Model file for the job. Use its own axes, mm. A direction names the side the tool comes from. Round coordinates to 2 decimals unless told otherwise and drop trailing zeros. Loops run counter-clockwise (first coordinate to the right, second up) from the corner with the lowest first, then second, coordinate; pieces in that order, holes last. Notation, with made-up numbers: M -26.75,-9.75 L -10.75,-9.75 A30 cw -10.75,21.25 Z; hole C 68,-36 d8. An arc over 180 degrees is marked long. Use a Markdown table: item, result. Add a question column.
Q1. Probe line 1 (Z direction, x = 0, y = 71); line 2 (X direction, y = 36.5, z = 0); line 3 (Z direction, x = 0, y = 34.5). List the from-to ranges inside material, lowest first. Write a range as from..to.
Q2. Cut at C-C (x = 53). State how many separate pieces and enclosed holes the cut face has, plus the area to 3 significant figures.
Q3. Cut at A-A (y = 71.5). Give the cut face in (x, z).
Q4. Cut at B-B (z = -59). Give the cut face in (x, y).
Q5. Tool access for faces 1 (the face through (2.1, 18, -25.1)), 2 (the face through (-17.35, 59.24, 29.33)), 3 (the face through (31, 59, 0)), 4 (the face through (-45.59, 7, -30.79)): list every direction of +Z, -Z, +X, -X, +Y, -Y with a clear straight run to the whole face (end or side of a thin tool).
Q6. Pin check, flat tips, straight feed: pin 1 (9 mm diameter, centred on x = 50.5, z = -31, fed in from +Y); pin 2 (1.5 mm diameter, centred on x = -27.5, y = 57, fed in from +Z); pin 3 (8 mm diameter, centred on x = 47.5, z = 0, fed in from +Y). Stop position of each tip, or through.
Q7. Mould opens along Z. For faces 5 (the face through (-31, 59, 0)), 6 (the face through (-46.235, 29.339, 16.238)), 7 (the face through (-56.465, 3.451, -28.308)), 8 (the face through (-17.119, 59.241, -29.665)) say: +Z half, -Z half, draft (parallel to the pull), parting line (faces both ways), or undercut.
from build123d import *

# Parameters (mm, degrees)
SKETCH1_R                               = 71
BOSS_EXTRUDE1_DEPTH                     = 18
BOSS_EXTRUDE2_DEPTH                     = 23
BOSS_EXTRUDE3_DEPTH                     = 37
CBORE_FOR_M5_HEX_HEAD_BOLT1_D           = 11
CBORE_FOR_M5_HEX_HEAD_BOLT1_CBORE_D     = 18
CBORE_FOR_M5_HEX_HEAD_BOLT1_CBORE_DEPTH = 11
CIRPATTERN1_COUNT                       = 6
F_10_0MM_DOWEL_HOLE1_D                  = 10
F_10_0MM_DOWEL_HOLE1_DEPTH              = 15
F_10_0MM_DOWEL_HOLE1_TIP                = 3.004303095
MIRROR2_OUTLINE_W                       = 2.5
MIRROR2_OUTLINE_H                       = 12.566951185
CUT_EXTRUDE1_REACH                      = 110.457
SKETCH17_R                              = 2.5


# Read off the part's stored shape, not the designer's step: Mirror2
with BuildPart() as part:
    # Sketch1 → Boss-Extrude1 (new body)
    with BuildSketch(Plane(origin=(0, 0, 0), x_dir=(1, 0, 0), z_dir=(0, 1, 0))):
        with Locations(Location((0, 0, 0), (0, 0, 270))):
            Circle(SKETCH1_R)
    extrude(amount=BOSS_EXTRUDE1_DEPTH)

    # Sketch2 → Boss-Extrude2 (add)
    with BuildSketch(Plane(origin=(0, 18, 0), x_dir=(1, 0, 0), z_dir=(0, 1, 0))):
        with BuildLine():
            Line((-50.50990002, 15), (-69.397406292, 15))
            ThreePointArc((-69.397406292, 15), (-71, 0), (-69.397406292, -15))
            Line((-69.397406292, -15), (-50.50990002, -15))
            ThreePointArc((-50.50990002, -15), (-46.181073535, -16.272350986), (-43.229193711, -19.684684685))
            ThreePointArc((-43.229193711, -19.684684685), (0, -47.5), (43.229193711, -19.684684685))
            ThreePointArc((43.229193711, -19.684684685), (46.181073535, -16.272350986), (50.50990002, -15))
            Line((50.50990002, -15), (69.397406292, -15))
            ThreePointArc((69.397406292, -15), (71, 0), (69.397406292, 15))
            Line((69.397406292, 15), (50.50990002, 15))
            ThreePointArc((50.50990002, 15), (46.181073535, 16.272350986), (43.229193711, 19.684684685))
            ThreePointArc((43.229193711, 19.684684685), (0, 47.5), (-43.229193711, 19.684684685))
            ThreePointArc((-43.229193711, 19.684684685), (-46.181073535, 16.272350986), (-50.50990002, 15))
        make_face()
    extrude(amount=BOSS_EXTRUDE2_DEPTH)

    # Sketch3 → Boss-Extrude3 (add)
    with BuildSketch(Plane(origin=(0, 41, 0), x_dir=(1, 0, 0), z_dir=(0, 1, 0))):
        with BuildLine():
            Line((9.027169873, -41.285714286), (25.440206006, -17.714285714))
            ThreePointArc((25.440206006, -17.714285714), (31, 0), (25.440206006, 17.714285714))
            Line((25.440206006, 17.714285714), (9.027169873, 41.285714286))
            ThreePointArc((9.027169873, 41.285714286), (0, 46), (-9.027169873, 41.285714286))
            Line((-9.027169873, 41.285714286), (-25.440206006, 17.714285714))
            ThreePointArc((-25.440206006, 17.714285714), (-31, 0), (-25.440206006, -17.714285714))
            Line((-25.440206006, -17.714285714), (-9.027169873, -41.285714286))
            ThreePointArc((-9.027169873, -41.285714286), (0, -46), (9.027169873, -41.285714286))
        make_face()
    extrude(amount=BOSS_EXTRUDE3_DEPTH)

    # CBORE for M5 Hex Head Bolt1 (through all)
    with Locations(Plane(origin=(0, 18, 59), x_dir=(0, 0, 1), z_dir=(0, 1, 0))):
        with Locations((0, 0)):
            cbore_for_m5_hex_head_bolt1 = CounterBoreHole(CBORE_FOR_M5_HEX_HEAD_BOLT1_D / 2, CBORE_FOR_M5_HEX_HEAD_BOLT1_CBORE_D / 2, CBORE_FOR_M5_HEX_HEAD_BOLT1_CBORE_DEPTH)

    # CirPattern1: CBORE for M5 Hex Head Bolt1 ×6 about axis
    cirpattern1_axis = Axis((0, 0, 0), (0, 1, 0))
    for i in range(1, CIRPATTERN1_COUNT):
        add(cbore_for_m5_hex_head_bolt1.rotate(cirpattern1_axis, i * 360 / CIRPATTERN1_COUNT), mode=Mode.SUBTRACT)

    # Ø10.0mm Dowel Hole1
    with Locations(Plane(origin=(0, 78, -35), x_dir=(0, 0, 1), z_dir=(0, 1, 0))):
        with Locations((0, 0), (70, 0)):
            Hole(F_10_0MM_DOWEL_HOLE1_D / 2, depth=F_10_0MM_DOWEL_HOLE1_DEPTH)
            with Locations((0, 0, -(F_10_0MM_DOWEL_HOLE1_DEPTH + F_10_0MM_DOWEL_HOLE1_TIP / 2))):  # 118° drill point
                Cone(0, F_10_0MM_DOWEL_HOLE1_D / 2, F_10_0MM_DOWEL_HOLE1_TIP, mode=Mode.SUBTRACT)

    # Sketch12 → Cut-Revolve3 (revolve, cut)
    with BuildSketch(Plane(origin=(0, 0, 0), x_dir=(0, 0, -1), z_dir=(1, 0, 0))):
        with BuildLine():
            Line((0, 0), (31, 0))
            Line((31, 0), (31, 18))
            Line((31, 18), (25, 18))
            Line((25, 18), (22.043106659, 29.03527618))
            ThreePointArc((22.043106659, 29.03527618), (20.61444907, 31.173413361), (18.179403354, 32))
            Line((18.179403354, 32), (11.248711306, 32))
            Line((11.248711306, 32), (11.248711306, 41))
            Line((11.248711306, 41), (23, 41))
            Line((23, 41), (23, 78))
            Line((23, 78), (0, 78))
            Line((0, 78), (0, 0))
        make_face()
    revolve(axis=Axis((0, 0, 0), (0, 1, 0)), mode=Mode.SUBTRACT)

    # Sketch13 → CBORE for M5 Hex Head Bolt2 (revolve, cut)
    with BuildSketch(Plane(origin=(-70.999948097, 18, -0.085850351), x_dir=(-0.001209159868286979, 0, 0.9999992689659393), z_dir=(0, 1, 0))):
        Polygon((0, 0), (0, 35.605163714), (6, 32), (6, 4), (10, 4), (10, 0), align=None)
    cbore_for_m5_hex_head_bolt2 = revolve(axis=Axis((-77.349943455, 18, -0.093528516), (0.9999992689659393, 0, 0.001209159868286979)), mode=Mode.SUBTRACT)

    # Mirror1: CBORE for M5 Hex Head Bolt2 across plane
    add(cbore_for_m5_hex_head_bolt2.mirror(Plane(origin=(0, 0, 0), x_dir=(0, 0, 1), z_dir=(1, 0, 0))), mode=Mode.SUBTRACT)

    # Sketch16 → Ø5.0mm Dowel Hole1 (revolve, cut)
    with BuildSketch(Plane(origin=(-70.999948097, 18, -0.085850351), x_dir=(-0.001209159868286979, 0, 0.9999992689659393), z_dir=(0, 1, 0))):
        Polygon((0, 0), (0, 72.501151548), (2.5, 70.999), (2.5, 0), align=None)
    revolve(axis=Axis((-77.349943455, 18, -0.093528516), (0.9999992689659393, 0, 0.001209159868286979)), mode=Mode.SUBTRACT)

    # Mirror2 outline → Mirror2 (revolve, cut)
    with BuildSketch(Plane(origin=(0, 18, 0), x_dir=(0, 1, 0), z_dir=(-0.0012091598682869803, 0, -0.9999992689659393))):
        with Locations((1.25, 30.613512241)):
            Rectangle(MIRROR2_OUTLINE_W, MIRROR2_OUTLINE_H)
        Polygon((2.5, -25.031211929), (2.5, -24.330096403), (2.439383393, -24.330096403), (2.439383393, -25.067634061), align=None)
    revolve(axis=Axis((0, 18, 0), (0.9999992689659393, 0, -0.0012091598682869803)), mode=Mode.SUBTRACT)

    # Sketch17 → Cut-Extrude1 (cut, up to next)
    with BuildSketch(Plane(origin=(0, 41, 0), x_dir=(1, 0, 0), z_dir=(0, 1, 0)), mode=Mode.PRIVATE) as cut_extrude1_sk1:
        with Locations(Location((-47.5, 0, 0), (0, 0, 270))):
            Circle(SKETCH17_R)
    cut_extrude1_tool1 = extrude(cut_extrude1_sk1.sketch, amount=-CUT_EXTRUDE1_REACH, mode=Mode.PRIVATE) & part.part
    # Sketch17 → Cut-Extrude1 (cut, up to next)
    with BuildSketch(Plane(origin=(0, 41, 0), x_dir=(1, 0, 0), z_dir=(0, 1, 0)), mode=Mode.PRIVATE) as cut_extrude1_sk2:
        with Locations(Location((47.5, 0, 0), (0, 0, 270))):
            Circle(SKETCH17_R)
    cut_extrude1_tool2 = extrude(cut_extrude1_sk2.sketch, amount=-CUT_EXTRUDE1_REACH, mode=Mode.PRIVATE) & part.part
    add(cut_extrude1_tool1.solids().sort_by_distance((-47.5, 41, 0))[0], mode=Mode.SUBTRACT)
    add(cut_extrude1_tool2.solids().sort_by_distance((47.5, 41, 0))[0], mode=Mode.SUBTRACT)


solid = part.part
Checked values:
| question | item | result |
|---|---|---|
| 1 | line 1 | z = -46..-40, -30..-23, 23..30, 40..46 |
| 1 | line 2 | x = -71..-50, -45..-11.25, 11.25..45, 50..71 |
| 1 | line 3 | z = -47.5..-11.25, 11.25..47.5 |
| 2 | separate pieces | 3 |
| 2 | enclosed holes | 1 |
| 2 | area | 1,750 mm^2 |
| 3 | outline | M -25.44,-17.71 L -9.03,-41.29 A11 ccw 9.03,-41.29 L 25.44,-17.71 A31 ccw 25.44,17.71 L 9.03,41.29 A11 ccw -9.03,41.29 L -25.44,17.71 A31 ccw Z; hole C 0,0 d46; hole C 0,-35 d10; hole C 0,35 d10 |
| 4 | outline | M -39.5,0 L -5.5,0 L -5.5,7 L -9,7 L -9,18 L -39.5,18 Z; M 5.5,0 L 39.5,0 L 39.5,18 L 9,18 L 9,7 L 5.5,7 Z |
| 5 | face 1 | -Y |
| 5 | face 2 | +Z, -X, +Y |
| 5 | face 3 | +X, +Y |
| 5 | face 4 | +Y |
| 6 | pin 1 | stops at y = 7 |
| 6 | pin 2 | stops at z = 15.67 |
| 6 | pin 3 | stops at y = 41 |
| 7 | face 5 | parting line |
| 7 | face 6 | +Z half |
| 7 | face 7 | undercut |
| 7 | face 8 | -Z half |
